Check sheet for the drawn part. Datum: minimum x, y, z corner. Units: mm. Give positions to 0.01 mm unless a question says otherwise; leave off trailing zeros. Order: outer loops, then holes, each group sorted by start corner. A loop starts at its lowest first (then second) coordinate and runs counter-clockwise, first axis right, second up. Notation, with made-up numbers: (21, 84) -> (52, 84) arc R21 ccw to (52, 111) -> close; hole circle Ø7 at (47.25, 26.25). An arc over 180 degrees is marked (long way). One line per question, with ' | ' between items. Start each with the question number.
Q1. Mould release check, pull along Y, two halves, no side actions. Record for the marked faces 1, 2 and 3: released by +Y, released by -Y, zero draft, split by the parting line, or undercut.
Q2. Section check A-A on y = 25.4. Record the cut outline in (x, z).
Q3. Material ranges on probe 1 along Y at (x, z) = (29, 3.5) (1 decimal); probe 2 along X at (y, z) = (24.5, 4.25) (1 decimal); probe 3 along X at (y, z) = (25.5, 8), recorded low to high. Write a range as [from, to].
Q4. Go/stop test with flat-tipped pins: pin 1 (2 mm diameter, centred on x = 23.5, z = 2.5, fed in from -Y); pin 2 (5 mm diameter, centred on x = 11.5, z = 2.5, fed in from +Y); pin 3 (12 mm diameter, centred on x = 19.5, y = 30.5, fed in from -Z); pin 4 (4 mm diameter, centred on y = 12.5, z = 10.5, fed in from +X). Record where each tip stops, or that it passes through.
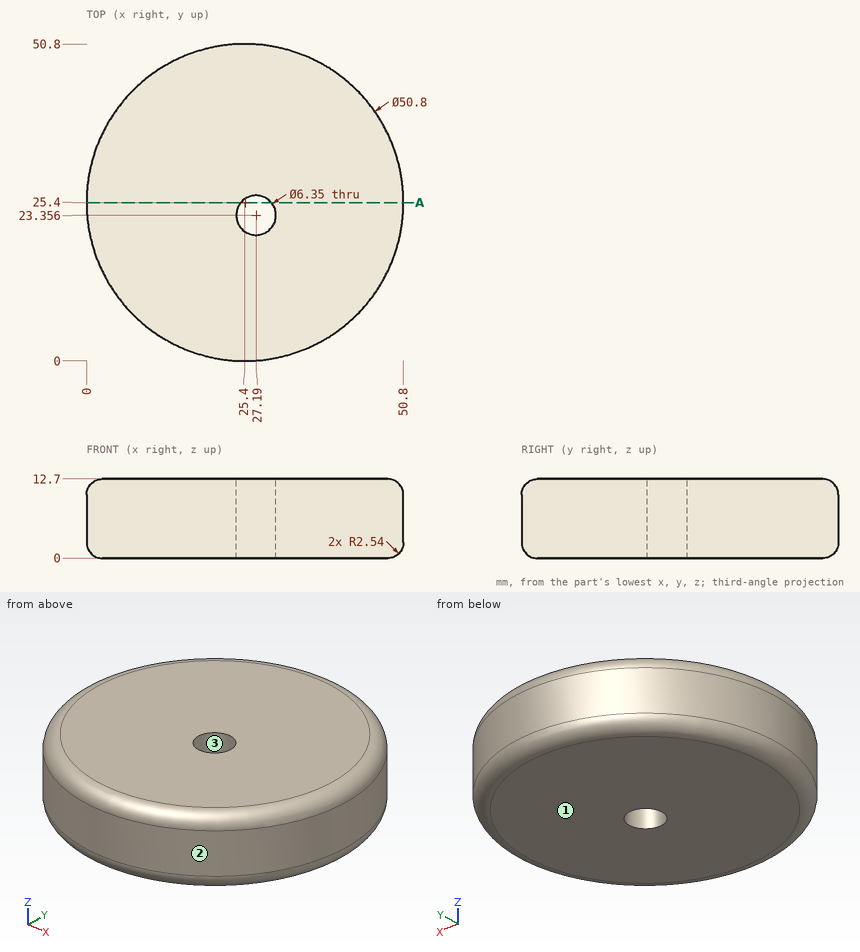
Filled in:
1) face 1: zero draft | face 2: split by the parting line | face 3: undercut
2) outline: (0, 2.54) arc R2.54 ccw to (2.54, 0) -> (24.76, 0) -> (24.76, 12.7) -> (2.54, 12.7) arc R2.54 ccw to (0, 10.16) -> close; (29.62, 0) -> (48.26, 0) arc R2.54 ccw to (50.8, 2.54) -> (50.8, 10.16) arc R2.54 ccw to (48.26, 12.7) -> (29.62, 12.7) -> close
3) probe 1: [0.3, 20.7], [26, 50.5] | probe 2: [0, 24.2], [30.2, 50.8] | probe 3: [0, 24.85], [29.53, 50.8]
4) pin 1: y = 0.02 | pin 2: y = 48.1 | pin 3: z = 0 | pin 4: x = 48.33
